Build history of the part. All positions in model axes, mm. A direction names the side the tool comes from. Give positions to 0.01 mm unless a question says otherwise; leave off trailing zeros. Order: outer loops, then holes, each group sorted by start corner. A loop starts at its lowest first (then second) coordinate and runs counter-clockwise, first axis right, second up. Notation, with made-up numbers: M 76.5,-31.75 L 116.5,-31.75 A13 cw 116.5,-22.75 Z; hole C 46.5,7.25 d11. An arc over 180 degrees is marked long. One line per item, written item: value.
from build123d import *

# Parameters (mm, degrees)
F0_W      = 150
F0_H      = 140
F1_DEPTH  = 2
F3_DEPTH  = 2.001
F5_DEPTH  = 2.001
F7_DEPTH  = 2.001
F8_R      = 50
F9_DEPTH  = 1
F11_DEPTH = 1


with BuildPart() as f1:
    # F0 (on Top) → F1 (new body)
    with BuildSketch(Plane.XY):
        Rectangle(F0_W, F0_H)
    extrude(amount=F1_DEPTH)

    # F2 (on face) → F3 (cut, through all)
    with BuildSketch(Plane.XY.offset(2)):
        Polygon((-75, 70), (-75, 41.5), (-46.5, 70), align=None)
        Polygon((-46.5, -70), (-75, -41.5), (-75, -70), align=None)
    extrude(amount=-F3_DEPTH, mode=Mode.SUBTRACT)

    # F4 (on face) → F5 (cut, through all)
    with BuildSketch(Plane.XY.offset(2)):
        with BuildLine():
            Line((-69.68, 9.5), (-75, 9.5))
            Line((-75, 9.5), (-75, -9.5))
            Line((-75, -9.5), (-69.68, -9.5))
            ThreePointArc((-69.68, -9.5), (-67.912233, -8.767767), (-67.18, -7))
            Line((-67.18, -7), (-67.18, 7))
            ThreePointArc((-67.18, 7), (-67.912233, 8.767767), (-69.68, 9.5))
        make_face()
    extrude(amount=-F5_DEPTH, mode=Mode.SUBTRACT)

    # F6 (on face) → F7 (cut, through all)
    with BuildSketch(Plane.XY.offset(2)):
        with BuildLine():
            Line((-28.031671, -70), (-15, -70))
            Line((-15, -70), (-16.416769, -66.495551))
            ThreePointArc((-16.416769, -66.495551), (-21.515836, -63.056988), (-26.614902, -66.495551))
            Line((-26.614902, -66.495551), (-28.031671, -70))
        make_face()
        with BuildLine():
            Line((-27.876137, 70), (-26.631231, 66.430881))
            ThreePointArc((-26.631231, 66.430881), (-21.438069, 62.742254), (-16.244907, 66.430881))
            Line((-16.244907, 66.430881), (-15, 70))
            Line((-15, 70), (-27.876137, 70))
        make_face()
    extrude(amount=-F7_DEPTH, mode=Mode.SUBTRACT)

    # F8 (on face) → F9 (join)
    with BuildSketch(Plane.XY.offset(2)):
        with Locations((-3.16, 0)):
            Circle(F8_R)
    extrude(amount=F9_DEPTH)

    # F10 (on face) → F11 (join)
    with BuildSketch(Plane.XY.offset(3)):
        with BuildLine():
            ThreePointArc((-2.16, -47.989582), (31.132856, -33.585711), (44.84, 0))
            ThreePointArc((44.84, 0), (31.132856, 33.585711), (-2.16, 47.989582))
            Line((-2.16, 47.989582), (-2.16, -47.989582))
        make_face()
        with BuildLine():
            Line((-4.16, -47.989582), (-4.16, 47.989582))
            ThreePointArc((-4.16, 47.989582), (-51.16, 0), (-4.16, -47.989582))
        make_face()
    extrude(amount=F11_DEPTH)


solid = f1.part
1) Drill centre lines: probe 1 along Z at (x, y) = (31, 34.5); probe 2 along X at (y, z) = (-1.5, 0.6); probe 3 along Z at (x, y) = (-51, 35). Where is each one in solid material? Low to high. Write a range as from..to.
Check values:
probe 1: 0..3
probe 2: -67.18..75
probe 3: 0..2
2) Saw through at B-B, the plane y = -18. Write the cut outline in (x, z).
Check values:
outline: M -75,0 L 75,0 L 75,2 L 43.49,2 L 43.49,3 L 41.34,3 L 41.34,4 L -2.16,4 L -2.16,3 L -4.16,3 L -4.16,4 L -47.66,4 L -47.66,3 L -49.81,3 L -49.81,2 L -75,2 Z
3) Pin check, flat tips, straight feed: pin 1 (0.8 mm diameter, centred on y = -22.5, z = 3.5, fed in from +X); pin 2 (0.6 mm diameter, centred on y = 1, z = 1, fed in from -X); pin 3 (1 mm diameter, centred on x = -72.5, z = 1, fed in from +Y). Stop position of each tip, or through.
Check values:
pin 1: x = 39.45
pin 2: x = -67.18
pin 3: y = 44.5
4) Saw through at D-D, the plane y = 25.5. Write the cut outline in (x, z), then the cut area to 3 significant figures.
Check values:
outline: M -75,0 L 75,0 L 75,2 L 39.85,2 L 39.85,3 L 37.51,3 L 37.51,4 L -2.16,4 L -2.16,3 L -4.16,3 L -4.16,4 L -43.83,4 L -43.83,3 L -46.17,3 L -46.17,2 L -75,2 Z
area: 465 mm^2
5) Tool access for faces 1 (the face through (49, 1, 2)), 2 (the face through (-51.15, 1.04, 3.49)), 3 (the face through (-1, 1, 0)): list every direction of +Z, -Z, +X, -X, +Y, -Y with a clear straight run to the whole face (end or side of a thin tool).
Check values:
face 1: +Z
face 2: +Z, -X
face 3: -Z, +X, -X, +Y, -Y
6) Saw through at A-A, the plane z = 1.3. Write the cut outline in (x, y), then the cut area to 3 significant figures.
Check values:
outline: M -75,-41.5 L -46.5,-70 L -28.03,-70 L -26.61,-66.5 A5.5 cw -16.42,-66.5 L -15,-70 L 75,-70 L 75,70 L -15,70 L -16.24,66.43 A5.5 cw -26.63,66.43 L -27.88,70 L -46.5,70 L -75,41.5 L -75,9.5 L -69.68,9.5 A2.5 cw -67.18,7 L -67.18,-7 A2.5 cw -69.68,-9.5 L -75,-9.5 Z
area: 19,900 mm^2
7) Mould opens along X. For faces 4 (the face through (44.53, 15.02, 2.49)), 5 (the face through (-60.6, -55.9, 1)), 6 (the face through (-21.424, -63.058, 1.014)) say: released by +X, released by -X, zero draft, split by the parting line, or undercut.
Check values:
face 4: split by the parting line
face 5: released by -X
face 6: undercut
8) Saw through at C-C, the plane x = -33. Write the cut outline in (y, z).
Check values:
outline: M -70,0 L 70,0 L 70,2 L 40.12,2 L 40.12,3 L 37.6,3 L 37.6,4 L -37.6,4 L -37.6,3 L -40.12,3 L -40.12,2 L -70,2 Z
